Could you check a few things on this drawing? It's one solid part, dimensions in mm from its lowest x, y, z. A direction names the side the tool comes from. Coordinates: 2 decimals unless noted, no trailing zeros. Write each loop counter-clockwise with the first axis right and the second up, starting at its lowest first coordinate (ties: lowest second). Pieces come first, ordered by that corner, then holes. Notation, with made-up numbers: M 79,-31.75 L 126,-31.75 A19 ccw 126,-26.75 Z; hole C 76,80 d9. An arc over 180 degrees is marked long. Use a Markdown table: item, result.
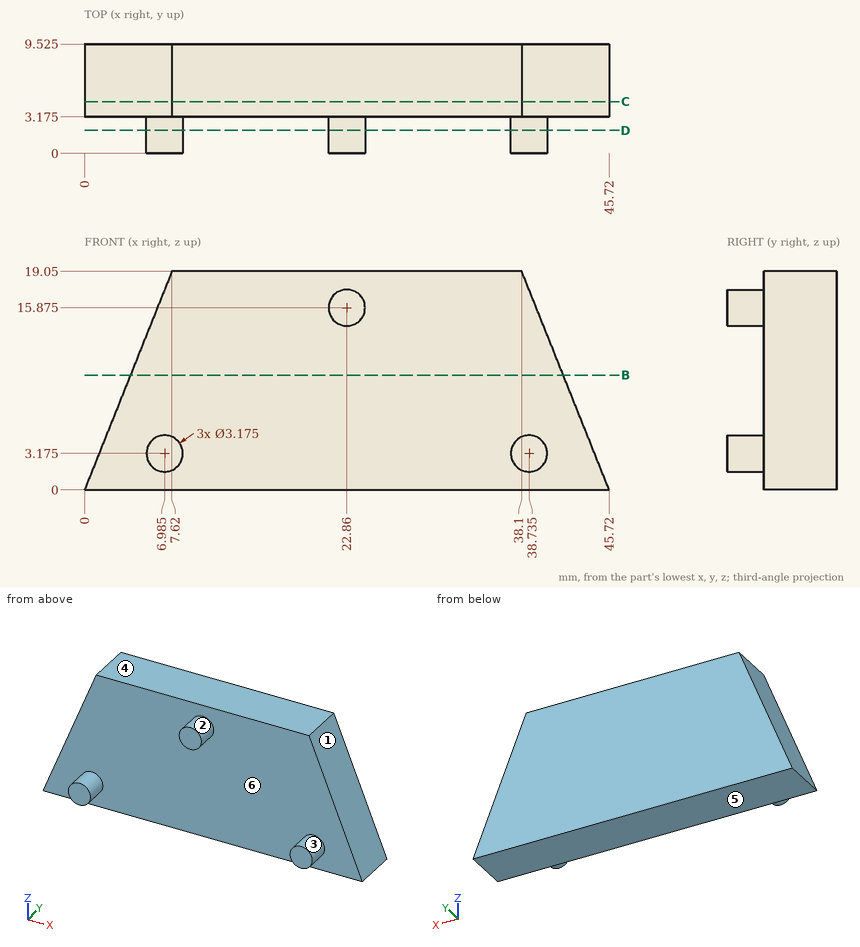
1. Will these pins go through, and if not, where does the flat tip stop? pin 1 Ø8 at (x, z) = (7.5, 11.5) entering from -Y (3 decimals); pin 2 Ø2 at (y, z) = (7.5, 2) entering from +X.
Answers follow:
| item | result |
|---|---|
| pin 1 | stops at y = 3.175 |
| pin 2 | stops at x = 45.32 |
2. We'd pull the mould along X, two halves only. Please class the marked faces 1, 2, 3 and 4: +X half, -X half, draft (parallel to the pull), parting line (faces both ways), or undercut.
Answers follow:
| item | result |
|---|---|
| face 1 | +X half |
| face 2 | parting line |
| face 3 | undercut |
| face 4 | draft |
3. Suppose I cut it at C-C on y = 4.5. Write out the boundary of the cut face in (x, z), and give its area (3 significant figures).
Answers follow:
| item | result |
|---|---|
| outline | M 0,0 L 45.72,0 L 38.1,19.05 L 7.62,19.05 Z |
| area | 726 mm2 |
4. Which directions (+Z, -Z, +X, -X, +Y, -Y) give clear straight access to the entire face, cutting with the end or side of a thin tool? Please do the marked faces 5 and 6.
Answers follow:
| item | result |
|---|---|
| face 5 | -Z, +X, -X, +Y, -Y |
| face 6 | -Y |
5. Suppose I cut it at D-D on y = 2. Write out the boundary of the cut face in (x, z) (1 decimal).
Answers follow:
| item | result |
|---|---|
| outline | C 7,3.2 d3.2; C 22.9,15.9 d3.2; C 38.7,3.2 d3.2 |
6. I need wall thicknesses on probe 1 along Y at (x, z) = (43, 3.25) (3 decimals); probe 2 along X at (y, z) = (8.75, 11.25); probe 3 along X at (y, z) = (5.75, 16.5). Which ranges of each line are inside material? Lowest first, please.
Answers follow:
| item | result |
|---|---|
| probe 1 | y = 3.175 to 9.525 |
| probe 2 | x = 4.5 to 41.22 |
| probe 3 | x = 6.6 to 39.12 |
7. Suppose I cut it at B-B on z = 10. Write out the boundary of the cut face in (x, y) (3 decimals), and give its area (3 significant figures).
Answers follow:
| item | result |
|---|---|
| outline | M 4,3.175 L 41.72,3.175 L 41.72,9.525 L 4,9.525 Z |
| area | 240 mm2 |
